Part print with two shaded views. Sizes in mm from the minimum x, y, z corner. A direction names the side the tool comes from. Coordinates: 2 decimals unless noted, no trailing zeros. Write each loop counter-clockwise with the first axis right and the second up, starting at its lowest first coordinate (ties: lowest second). Pieces come first, ordered by that corner, then holes. Notation, with made-up numbers: (-6.75, -26) - (30.25, -26) arc R23 cw to (30.25, 6) - close; hole circle Ø5 at (53.5, 85.5). An arc over 180 degrees is marked (long way). One line per question, with ' | ' between items. Start each with the question number.
1. Probe line 1 (X direction, y = 66, z = 45); line 2 (Z direction, x = 18.5, y = 37.5); line 3 (Y direction, x = 50, z = 37) (1 decimal). List the from-to ranges inside material, lowest first.
2. Two-plate mould, pull along X, no slides. Class the marked faces 1, 2 and 3: +X half, -X half, draft (parallel to the pull), parting line (faces both ways), or undercut.
3. Band-saw the part on D-D, the plane y = 17. Write the cut outline in (x, z), then the cut area to 3 significant figures.
4. Band-saw the part on C-C, the plane x = 39.5. Write the cut outline in (y, z), then the cut area to 3 significant figures.
5. Flat gauge pins, fed straight in: P1, Ø12, axis at x = 33, z = 66.5, coming from the -Y side; P2, Ø10, axis at y = 21, z = 21.5, coming from the -X side; P3, Ø5, axis at x = 41, y = 55.5, coming from the +Z side. Where does each tip first touch, or does it go through?
6. Which spindle directions (+Z, -Z, +X, -X, +Y, -Y) get a long thin tool onto all of the face, cutting with end or side? Do the marked faces 4, 5 and 6. Say none if no direction does.
7. Band-saw the part on A-A, the plane y = 37.5. Write the cut outline in (x, z).
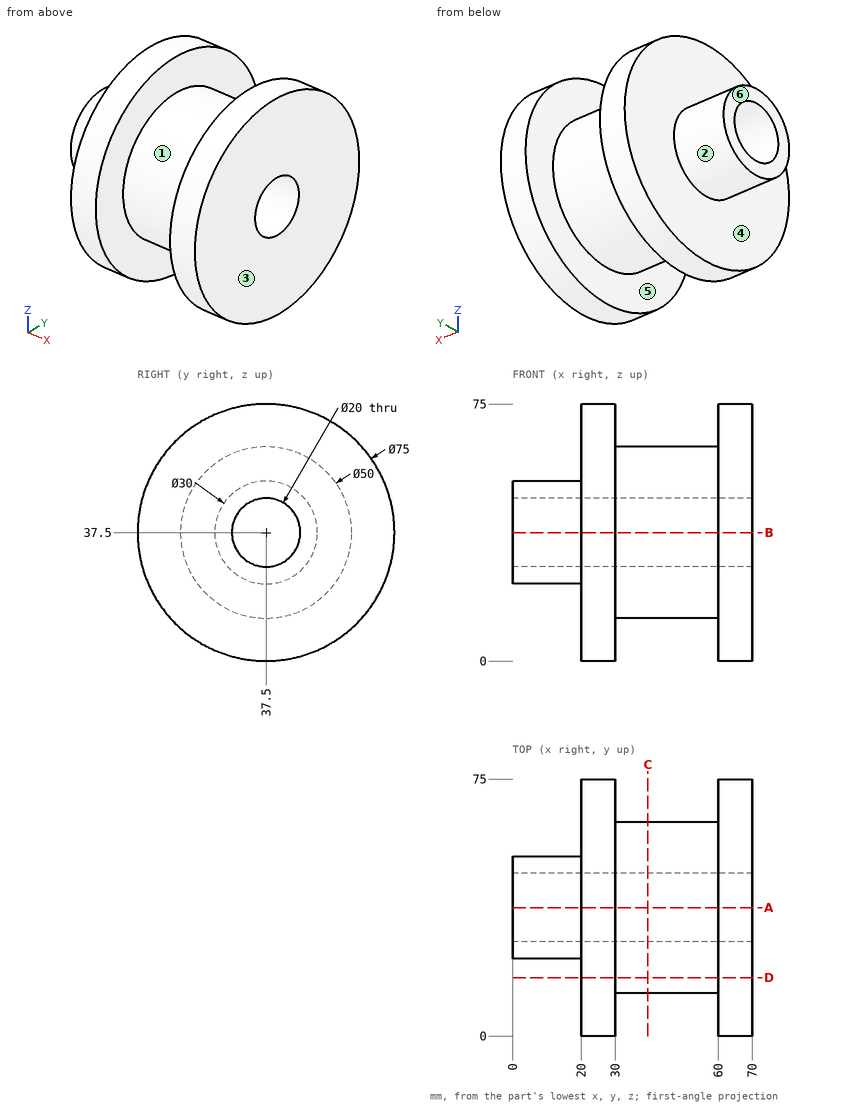
Filled in:
1) line 1: x = 20 to 30, 60 to 70 | line 2: z = 22.5 to 27.5, 47.5 to 52.5 | line 3: y = 12.5 to 27.5, 47.5 to 62.5
2) face 1: undercut | face 2: draft | face 3: +X half
3) outline: (20, 6.1) - (30, 6.1) - (30, 23.19) - (60, 23.19) - (60, 6.1) - (70, 6.1) - (70, 68.9) - (60, 68.9) - (60, 51.81) - (30, 51.81) - (30, 68.9) - (20, 68.9) - close | area: 2,110 mm²
4) outline: circle Ø50 at (37.5, 37.5); hole circle Ø20 at (37.5, 37.5) | area: 1,650 mm²
5) P1: stops at y = 8.52 | P2: stops at x = 20 | P3: stops at z = 57.12
6) face 4: -X | face 5: none | face 6: +Z, -Z, -X, +Y, -Y
7) outline: (0, 22.5) - (20, 22.5) - (20, 0) - (30, 0) - (30, 12.5) - (60, 12.5) - (60, 0) - (70, 0) - (70, 27.5) - (0, 27.5) - close; (0, 47.5) - (70, 47.5) - (70, 75) - (60, 75) - (60, 62.5) - (30, 62.5) - (30, 75) - (20, 75) - (20, 52.5) - (0, 52.5) - close
